The listing builds one solid part. Answer for the finished solid, in the listing's coordinates (mm). A direction names the side the tool comes from. Give positions to 0.01 mm unless a question says otherwise; leave off trailing zeros. Order: outer loops, then holes, each group sorted by start corner. A loop starts at its lowest first (then second) coordinate and runs counter-clockwise, first axis right, second up. Notation, with made-up numbers: (34.25, 10.5) - (90.25, 10.5) arc R21 cw to (90.25, 34.5) - close; hole circle Ø2 at (-12, -15). An arc over 180 degrees is marked (long way). Use a Markdown table: item, result. Add a question column.
1) The mould has two halves that part along X. Classify faces 5 (the face through (27.13, -8, 0.69)), 6 (the face through (3, -0.6, -2)), 7 (the face through (2.45, -14, -13)), 8 (the face through (-2.45, -14, -22)): released by +X, released by -X, zero draft, split by the parting line, or undercut.
2) For faces 1 (the face through (2.45, -14, -22)), 2 (the face through (10, -7, -16)), 3 (the face through (23.99, -4.06, -7.15)), 4 (the face through (21, -14, 2.45)), determine the directions among +Z, -Z, +X, -X, +Y, -Y from which every point of the face is accessible in a straight line to the end or side of a thin tool.
3) Find section A-A, the plane y = -1.5. State how many separate pieces and enclosed holes the cut face has, plus the area to 3 significant figures.
4) Find section D-D, the plane x = 21.5. Determine the outline of the cut face in (y, z), plus the area to 3 significant figures.
5) Straight lines are drawn through the part: line 1 (X direction, y = -11, z = -17); line 2 (Y direction, x = -2.5, z = -2.5); line 3 (Z direction, x = 22, y = -9.5). For each, find the intervals that lie inside material, in ascending order.
6) Find section B-B, the plane x = 33. Determine the outline of the cut face in (y, z).
7) Flat-ended cylindrical pins translate along their axes: pin 1 (1.1 mm diameter, centred on y = -14, z = 0.5, fed in from -X); pin 2 (10 mm diameter, centred on x = 29, z = -9.5, fed in from -Y); pin 3 (8 mm diameter, centred on x = 8.5, y = -12.5, fed in from -Z). Find the tip coordinate at first contact, or state that the pin passes through.
from build123d import *

# Parameters (mm, degrees)
BOSS_EXTRUDE1_DEPTH                             = 13.5
BOSS_EXTRUDE2_START                             = -13.5
SKETCH1_3_W                                     = 16.5
SKETCH1_3_H                                     = 4.9
BOSS_EXTRUDE2_DEPTH                             = 1
BOSS_EXTRUDE3_DEPTH                             = 0.6
CSK_FOR_M5_FLAT_HEAD_MACHINE_SCREW1_D           = 5.3
CSK_FOR_M5_FLAT_HEAD_MACHINE_SCREW1_CSINK_D     = 10.4
CSK_FOR_M5_FLAT_HEAD_MACHINE_SCREW1_CSINK_ANGLE = 90
BOSS_EXTRUDE4_START                             = -8
SKETCH1_5_W                                     = 12
SKETCH1_5_H                                     = 7.55
SKETCH1_5_H_2                                   = 4.9
BOSS_EXTRUDE4_DEPTH                             = 5.5
BOSS_EXTRUDE5_START                             = -13.5
SKETCH1_6_W                                     = 12
SKETCH1_6_H                                     = 4.9
BOSS_EXTRUDE5_DEPTH                             = 1
CSK_FOR_M5_FLAT_HEAD_MACHINE_SCREW2_D           = 5.3
CSK_FOR_M5_FLAT_HEAD_MACHINE_SCREW2_CSINK_D     = 10.4
CSK_FOR_M5_FLAT_HEAD_MACHINE_SCREW2_CSINK_ANGLE = 90
FILLET1_R                                       = 10
FILLET2_R                                       = 5
CUT_EXTRUDE1_DEPTH                              = 8
CHAMFER1_SIZE                                   = 1


with BuildPart() as part:
    # Sketch1 → Boss-Extrude1 (new body)
    with BuildSketch(Plane(origin=(0, 0, 0), x_dir=(1, 0, 0), z_dir=(0, 1, 0))):
        with BuildLine():
            Line((-1.919417382, -1.919417382), (-10, -10))
            Line((-10, -10), (27, -10))
            Line((27, -10), (27, -2.45))
            Line((27, -2.45), (10.5, -2.45))
            Line((10.5, -2.45), (10.5, 2.45))
            Line((10.5, 2.45), (18.900480814, 2.45))
            ThreePointArc((18.900480814, 2.45), (21.474998844, 5.099879794), (24.1, 2.5))
            ThreePointArc((24.1, 2.5), (24.099879794, 2.474998844), (24.099519186, 2.45))
            Line((24.099519186, 2.45), (27, 2.45))
            Line((27, 2.45), (27, 10))
            Line((27, 10), (10, 10))
            Line((10, 10), (6.919417382, 6.919417382))
            ThreePointArc((6.919417382, 6.919417382), (8.274247078, 4.891771452), (8.75, 2.5))
            ThreePointArc((8.75, 2.5), (4.891771452, -3.274247078), (-1.919417382, -1.919417382))
        make_face()
        with BuildLine():
            Line((10.5, -2.45), (27, -2.45))
            Line((27, -2.45), (27, 2.45))
            Line((27, 2.45), (24.099519186, 2.45))
            ThreePointArc((24.099519186, 2.45), (21.5, -0.1), (18.900480814, 2.45))
            Line((18.900480814, 2.45), (10.5, 2.45))
            Line((10.5, 2.45), (10.5, -2.45))
        make_face()
        with BuildLine():
            ThreePointArc((18.900480814, 2.45), (21.5, -0.1), (24.099519186, 2.45))
            Line((24.099519186, 2.45), (18.900480814, 2.45))
        make_face()
        with BuildLine():
            Line((18.900480814, 2.45), (24.099519186, 2.45))
            ThreePointArc((24.099519186, 2.45), (24.099879794, 2.474998844), (24.1, 2.5))
            ThreePointArc((24.1, 2.5), (21.474998844, 5.099879794), (18.900480814, 2.45))
        make_face()
    extrude(amount=-BOSS_EXTRUDE1_DEPTH)

    # Sketch1<3> → Boss-Extrude2 (add)
    with BuildSketch(Plane(origin=(0, 0, 0), x_dir=(1, 0, 0), z_dir=(0, 1, 0)).offset(BOSS_EXTRUDE2_START)):
        with Locations((18.75, 0)):
            Rectangle(SKETCH1_3_W, SKETCH1_3_H)
    extrude(amount=-BOSS_EXTRUDE2_DEPTH)

    # Sketch1<4> → Boss-Extrude3 (add)
    with BuildSketch(Plane(origin=(0, 0, 0), x_dir=(1, 0, 0), z_dir=(0, 1, 0))):
        with BuildLine():
            Line((6.919417382, 6.919417382), (-1.919417382, -1.919417382))
            ThreePointArc((-1.919417382, -1.919417382), (4.891771452, -3.274247078), (8.75, 2.5))
            ThreePointArc((8.75, 2.5), (8.274247078, 4.891771452), (6.919417382, 6.919417382))
        make_face()
    extrude(amount=-BOSS_EXTRUDE3_DEPTH)

    # Mirror1: part across plane


with BuildPart() as part_1:
    add(part.part)
    add(part.part.mirror(Plane(origin=(0, -13.5, 0), x_dir=(-0.7071067811865465, 0, 0.7071067811865486), z_dir=(0.7071067811865488, 0, 0.7071067811865464))))

    # CSK for M5 Flat Head Machine Screw1 (through all)
    with Locations(Plane(origin=(0, 0, 0), x_dir=(1, 0, 0), z_dir=(0, 1, 0))):
        with Locations((0, 17)):
            CounterSinkHole(CSK_FOR_M5_FLAT_HEAD_MACHINE_SCREW1_D / 2, CSK_FOR_M5_FLAT_HEAD_MACHINE_SCREW1_CSINK_D / 2, counter_sink_angle=CSK_FOR_M5_FLAT_HEAD_MACHINE_SCREW1_CSINK_ANGLE)

    # Sketch1<5> → Boss-Extrude4 (add)
    with BuildSketch(Plane(origin=(0, 0, 0), x_dir=(1, 0, 0), z_dir=(0, 1, 0)).offset(BOSS_EXTRUDE4_START)):
        with Locations((33, 6.225)):
            Rectangle(SKETCH1_5_W, SKETCH1_5_H)
        with Locations((33, 0)):
            Rectangle(SKETCH1_5_W, SKETCH1_5_H_2)
        with Locations((33, -6.225)):
            Rectangle(SKETCH1_5_W, SKETCH1_5_H)
    extrude(amount=-BOSS_EXTRUDE4_DEPTH)

    # Sketch1<6> → Boss-Extrude5 (add)
    with BuildSketch(Plane(origin=(0, 0, 0), x_dir=(1, 0, 0), z_dir=(0, 1, 0)).offset(BOSS_EXTRUDE5_START)):
        with Locations((33, 0)):
            Rectangle(SKETCH1_6_W, SKETCH1_6_H)
    extrude(amount=-BOSS_EXTRUDE5_DEPTH)

    # CSK for M5 Flat Head Machine Screw2 (through all)
    with Locations(Plane(origin=(0, -8, 0), x_dir=(1, 0, 0), z_dir=(0, 1, 0))):
        with Locations((33, 0)):
            CounterSinkHole(CSK_FOR_M5_FLAT_HEAD_MACHINE_SCREW2_D / 2, CSK_FOR_M5_FLAT_HEAD_MACHINE_SCREW2_CSINK_D / 2, counter_sink_angle=CSK_FOR_M5_FLAT_HEAD_MACHINE_SCREW2_CSINK_ANGLE)

    # Fillet1
    fillet1_edges = [part_1.edges().sort_by_distance(p)[0] for p in [
        (-10, -6.75, -27),
        (10, -6.75, -27),
        (39, -10.75, -10),
        (39, -10.75, 10),
        (27, -4, -10),
        (27, -4, 10),
        (-10, -6.75, 10),
    ]]
    fillet(fillet1_edges, radius=FILLET1_R - 0.0001)  # a hair under: the kernel refuses the full size

    # Fillet2
    fillet2_edges = [part_1.edges().sort_by_distance(p)[0] for p in [
        (10, -6.75, -10),
    ]]
    fillet(fillet2_edges, radius=FILLET2_R)

    # Sketch1<8> → Cut-Extrude1 (cut)
    with BuildSketch(Plane(origin=(0, 0, 0), x_dir=(1, 0, 0), z_dir=(0, 1, 0))):
        with BuildLine():
            ThreePointArc((18.900480814, 2.45), (21.5, -0.1), (24.099519186, 2.45))
            Line((24.099519186, 2.45), (18.900480814, 2.45))
        make_face()
        with BuildLine():
            Line((18.900480814, 2.45), (24.099519186, 2.45))
            ThreePointArc((24.099519186, 2.45), (24.099879794, 2.474998844), (24.1, 2.5))
            ThreePointArc((24.1, 2.5), (21.474998844, 5.099879794), (18.900480814, 2.45))
        make_face()
    extrude(amount=-CUT_EXTRUDE1_DEPTH, mode=Mode.SUBTRACT)

    # Chamfer1
    chamfer1_edges = [part_1.edges().sort_by_distance(p)[0] for p in [
        (24.099519186, -8, -2.55),
    ]]
    chamfer(chamfer1_edges, length=CHAMFER1_SIZE)


solid = part_1.part
The answers:
| question | item | result |
|---|---|---|
| 1 | face 5 | zero draft |
| 1 | face 6 | undercut |
| 1 | face 7 | released by +X |
| 1 | face 8 | released by -X |
| 2 | face 1 | +Z, -Z, +X, -Y |
| 2 | face 2 | -Z, +X, +Y, -Y |
| 2 | face 3 | -Z, +X, +Y |
| 2 | face 4 | +Z, +X, -X, -Y |
| 3 | separate pieces | 1 |
| 3 | enclosed holes | 3 |
| 3 | area | 791 mm2 |
| 4 | outline | (-14.5, -2.45) - (-13.5, -2.45) - (-13.5, -10) - (-8, -10) - (-8, -8.93) - (0, -8.93) - (0, -5.1) - (-7, -5.1) - (-8, -4.1) - (-8, -0.9) - (-7, 0.1) - (0, 0.1) - (0, 8.93) - (-8, 8.93) - (-8, 10) - (-13.5, 10) - (-13.5, 2.45) - (-14.5, 2.45) - close |
| 4 | area | 217 mm2 |
| 5 | line 1 | -10 to -2.65, 2.65 to 10 |
| 5 | line 2 | -0.6 to 0 |
| 5 | line 3 | -10 to 10 |
| 6 | outline | (-13.5, -9.17) - (-8, -9.17) - (-8, -5.2) - (-10.55, -2.65) - (-13.5, -2.65) - close; (-13.5, 2.65) - (-10.55, 2.65) - (-8, 5.2) - (-8, 9.17) - (-13.5, 9.17) - close |
| 7 | pin 1 | x = -10 |
| 7 | pin 2 | y = -13.5 |
| 7 | pin 3 | z = -25.93 |
